Verification items for the finished model (mm, model axes). Face numbers are marked on the shaded views. A direction names the side the tool comes from. Coordinates: 2 decimals unless noted, no trailing zeros. Order: outer loops, then holes, each group sorted by start corner. A loop starts at its lowest first (then second) coordinate and runs counter-clockwise, first axis right, second up. Notation, with made-up numbers: M -5,-24 L 1,-24 A27 ccw 1,15 Z; hole C 64.25,45 d4. An arc over 180 degrees is marked long. Return JSON: item names as keys, results as strings. Group by question number.
1. Set-up check for the marked faces 1, 2, 3 and 4: record each of +Z, -Z, +X, -X, +Y, -Y from which the full face is reachable in a straight line by a thin tool's end or side.
2. Section check A-A, the plane y = 0. Record the cut outline in (x, z).
3. Material ranges on line 1 along X through (y, z) = (0, -2.2); line 2 along X through (y, z) = (-6.25, 11.25); line 3 along Y through (x, z) = (-9.5, 7.75), recorded low to high.
4. Section check C-C, the plane z = 3.5. Record the cut outline in (x, y).
5. Section check B-B, the plane x = 27.5. Record the cut outline in (y, z).
6. Gauge pin test, flat ends, axial feed: pin 1 (7 mm diameter, centred on x = -26.5, y = 1.5, fed in from +Z); pin 2 (6 mm diameter, centred on y = 4.5, z = 9, fed in from -X); pin 3 (6 mm diameter, centred on y = -5.5, z = 6, fed in from +X). Record the tip position at first contact, or that the pin passes through.
7. Section check D-D, the plane x = 1. Record the cut outline in (y, z).
8. Mould release check, pull along Y, two halves, no side actions. Record for the marked faces 5, 6, 7 and 8: +Y half, -Y half, draft (parallel to the pull), parting line (faces both ways), or undercut.
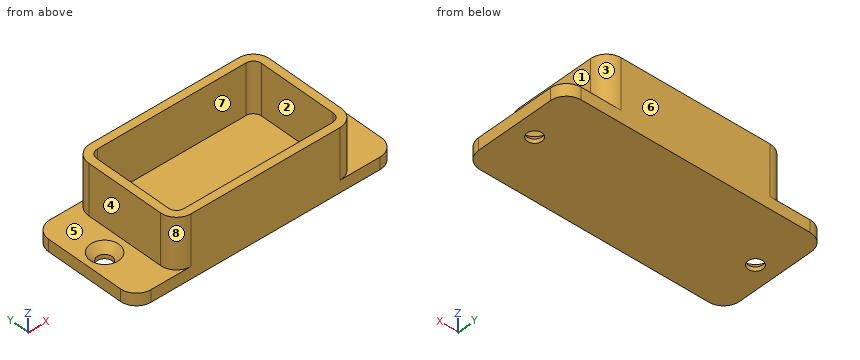
```python
from build123d import *

# Parameters (mm, degrees)
WALLS_SKETCH_W                 = 45
WALLS_SKETCH_H                 = 27.5
WALLS_SKETCH_W_2               = 41
WALLS_SKETCH_H_2               = 23.5
WALLS_EXTRUDE_DEPTH            = 15.5
BASE_SKETCH_W                  = 65
BASE_SKETCH_H                  = 27.5
BASE_EXTRUDE_DEPTH             = 3
NO_6_MOUNTING_HOLES_AT_2_COUNT = 2
NO_6_MOUNTING_HOLES_AT_2_PITCH = 55
TAB_FILLETS_R                  = 4
INSIDE_CORNER_FILLETS_R        = 2
OUTSIDE_CORNER_FILLETS_R       = 4


with BuildPart() as part:
    # Walls Sketch → Walls Extrude (new body)
    with BuildSketch(Plane.XY.offset(-2.5)):
        Rectangle(WALLS_SKETCH_W, WALLS_SKETCH_H)
        Rectangle(WALLS_SKETCH_W_2, WALLS_SKETCH_H_2, mode=Mode.SUBTRACT)
    extrude(amount=WALLS_EXTRUDE_DEPTH)

    # Base Sketch → Base Extrude (add)
    with BuildSketch(Plane.XY.offset(-2.5)):
        Rectangle(BASE_SKETCH_W, BASE_SKETCH_H)
    extrude(amount=BASE_EXTRUDE_DEPTH)

    # No. 6 Mounting Holes Profile Sketch → No. 6 Mounting Holes (revolve, cut)
    with BuildSketch(Plane(origin=(-27.5, 0, 0.5), x_dir=(0, -1, 0), z_dir=(1, 0, 0))):
        Polygon((0, 0), (0, 3), (1.8288, 3), (1.8288, 1.972306634), (3.5433, 0), align=None)
    no_6_mounting_holes = revolve(axis=Axis((-27.5, 0, 6.85), (0, 0, -1)), mode=Mode.SUBTRACT)

    # No. 6 Mounting Holes at 2: No. 6 Mounting Holes ×2
    with Locations(*[(i * NO_6_MOUNTING_HOLES_AT_2_PITCH, 0, 0) for i in range(1, NO_6_MOUNTING_HOLES_AT_2_COUNT)]):
        add(no_6_mounting_holes, mode=Mode.SUBTRACT)

    # Tab Fillets
    tab_fillets_edges = [part.edges().sort_by_distance(p)[0] for p in [
        (-32.5, -13.75, -1),
        (32.5, 13.75, -1),
        (-32.5, 13.75, -1),
        (32.5, -13.75, -1),
    ]]
    fillet(tab_fillets_edges, radius=TAB_FILLETS_R)

    # Inside Corner Fillets
    inside_corner_fillets_edges = [part.edges().sort_by_distance(p)[0] for p in [
        (-20.5, -11.75, 6.75),
        (20.5, -11.75, 6.75),
        (-20.5, 11.75, 6.75),
        (20.5, 11.75, 6.75),
    ]]
    fillet(inside_corner_fillets_edges, radius=INSIDE_CORNER_FILLETS_R)

    # Outside Corner Fillets
    outside_corner_fillets_edges = [part.edges().sort_by_distance(p)[0] for p in [
        (22.5, -13.75, 6.75),
        (-22.5, -13.75, 6.75),
        (-22.5, 13.75, 6.75),
        (22.5, 13.75, 6.75),
    ]]
    fillet(outside_corner_fillets_edges, radius=OUTSIDE_CORNER_FILLETS_R)


solid = part.part
```
Answers follow:
{
 "1": {"face 1": "+Z, +X, +Y, -Y", "face 2": "+Z", "face 3": "+Z, +X, +Y", "face 4": "+Z, -X, +Y, -Y"},
 "2": {"outline": "M -32.5,-2.5 L -29.33,-2.5 L -29.33,-1.47 L -31.04,0.5 L -32.5,0.5 Z; M -25.67,-2.5 L 25.67,-2.5 L 25.67,-1.47 L 23.96,0.5 L 22.5,0.5 L 22.5,13 L 20.5,13 L 20.5,0.5 L -20.5,0.5 L -20.5,13 L -22.5,13 L -22.5,0.5 L -23.96,0.5 L -25.67,-1.47 Z; M 29.33,-2.5 L 32.5,-2.5 L 32.5,0.5 L 31.04,0.5 L 29.33,-1.47 Z"},
 "3": {"line 1": "-32.5 to -29.33, -25.67 to 25.67, 29.33 to 32.5", "line 2": "-22.5 to -20.5, 20.5 to 22.5", "line 3": "-13.75 to -11.75, 11.75 to 13.75"},
 "4": {"outline": "M -22.5,-9.75 A4 ccw -18.5,-13.75 L 18.5,-13.75 A4 ccw 22.5,-9.75 L 22.5,9.75 A4 ccw 18.5,13.75 L -18.5,13.75 A4 ccw -22.5,9.75 Z; hole M -20.5,-9.75 A2 ccw -18.5,-11.75 L 18.5,-11.75 A2 ccw 20.5,-9.75 L 20.5,9.75 A2 ccw 18.5,11.75 L -18.5,11.75 A2 ccw -20.5,9.75 Z"},
 "5": {"outline": "M -13.75,-2.5 L -1.83,-2.5 L -1.83,-1.47 L -3.54,0.5 L -13.75,0.5 Z; M 1.83,-2.5 L 13.75,-2.5 L 13.75,0.5 L 3.54,0.5 L 1.83,-1.47 Z"},
 "6": {"pin 1": "z = 0.5", "pin 2": "x = -22.5", "pin 3": "x = 22.5"},
 "7": {"outline": "M -13.75,-2.5 L 13.75,-2.5 L 13.75,13 L 11.75,13 L 11.75,0.5 L -11.75,0.5 L -11.75,13 L -13.75,13 Z"},
 "8": {"face 5": "draft", "face 6": "+Y half", "face 7": "undercut", "face 8": "-Y half"}
}
